```python
from build123d import *

# Parameters (mm, degrees)
CHAMFER1_SIZE      = 2.54
CUT_EXTRUDE1_DEPTH = 111.185656707
SKETCH6_R          = 58.335249529
SKETCH6_R_2        = 20.235249529
CUT_EXTRUDE2_DEPTH = 5.08
CUT_EXTRUDE3_START = -5.08
SKETCH7_R          = 58.335249529
SKETCH7_R_2        = 20.235249529
CUT_EXTRUDE3_DEPTH = 5.08
FILLET15_R         = 7.62


with BuildPart() as part:
    # Sketch2 → Revolve1 (revolve)
    with BuildSketch(Plane.YZ, mode=Mode.PRIVATE) as revolve1_sk:
        Polygon((8.128, 0), (8.128, 19.304), (76.708, 19.304), (76.708, 12.065), (64.008, 12.065), (64.008, 7.239), (76.708, 7.239), (76.708, 0), align=None)
    revolve(revolve1_sk.sketch.rotate(Axis((0, 0, 0), (0, 0, 1)), 90), axis=Axis((0, 0, 0), (0, 0, 1)))

    # Chamfer1
    chamfer1_edges = [part.edges().sort_by_distance(p)[0] for p in [
        (76.708, 0, 0),
        (76.708, 0, 7.239),
        (76.708, 0, 12.065),
        (76.708, 0, 19.304),
    ]]
    chamfer(chamfer1_edges, length=CHAMFER1_SIZE)

    # Sketch5 → Cut-Extrude1 (cut, through all)
    with BuildSketch(Plane(origin=(0, 0, 0), x_dir=(1, 0, 0), z_dir=(0, 0, -1))):
        with BuildLine():
            Line((-58.42, 0), (-20.32, 0))
            ThreePointArc((-20.32, 0), (-13.061444229, 15.566023084), (3.52853097, 20.011293541))
            Line((3.52853097, 20.011293541), (10.144526539, 57.532468931))
            ThreePointArc((10.144526539, 57.532468931), (-37.551652158, 44.752316367), (-58.42, 0))
        make_face()
        with BuildLine():
            Line((29.21, -50.593204089), (10.16, -17.597636205))
            ThreePointArc((10.16, -17.597636205), (-6.949849312, -19.094554054), (-19.094554054, -6.949849312))
            Line((-19.094554054, -6.949849312), (-54.896842906, -19.980816773))
            ThreePointArc((-54.896842906, -19.980816773), (-19.980816773, -54.896842906), (29.21, -50.593204089))
        make_face()
        with BuildLine():
            Line((15.5725915, -12.921289312), (44.68739374, -37.497175605))
            ThreePointArc((44.68739374, -37.497175605), (57.44900601, 10.129809775), (29.167624765, 50.519808029))
            Line((29.167624765, 50.519808029), (10.117624765, 17.524240144))
            ThreePointArc((10.117624765, 17.524240144), (19.918066395, 3.568746925), (15.5725915, -12.921289312))
        make_face()
    extrude(amount=-CUT_EXTRUDE1_DEPTH, mode=Mode.SUBTRACT)

    # Sketch6 → Cut-Extrude2 (cut)
    with BuildSketch(Plane(origin=(0, 0, 0), x_dir=(1, 0, 0), z_dir=(0, 0, -1))):
        Circle(SKETCH6_R)
        with Locations(Location((0, 0, 0), (0, 0, 60))):
            Circle(SKETCH6_R_2, mode=Mode.SUBTRACT)
    extrude(amount=-CUT_EXTRUDE2_DEPTH, mode=Mode.SUBTRACT)

    # Sketch7 → Cut-Extrude3 (cut)
    with BuildSketch(Plane(origin=(0, 0, 19.304), x_dir=(0, -1, 0), z_dir=(0, 0, 1)).offset(CUT_EXTRUDE3_START)):
        Circle(SKETCH7_R)
        with Locations(Location((0, 0, 0), (0, 0, 90))):
            Circle(SKETCH7_R_2, mode=Mode.SUBTRACT)
    extrude(amount=CUT_EXTRUDE3_DEPTH, mode=Mode.SUBTRACT)

    # Fillet15
    # the kernel refuses this fillet: 7.62 mm, written as the material it adds along each edge
    with BuildSketch(Plane(origin=(10.16, 17.597636205, 5.08), x_dir=(-0.9266160044504649, 0.3760090162433024, 0), z_dir=(0, 0, 1)), Plane(origin=(-20.32, 0, 5.08), x_dir=(0.13767464210654276, -0.9904775075289874, 0), z_dir=(0, 0, 1))) as fillet15_piece_1:
        with BuildLine():
            CenterArc((6.644178228, -7.547438607), FILLET15_R, 97.913310066, 74.173379868)
            Line((-0.903260379, -6.498357835), (0, 0))
            ThreePointArc((0, 0), (2.797548728, -0.193497047), (5.595097455, 0))
        make_face()
    extrude(amount=9.144)
    with BuildSketch(Plane(origin=(-19.094554054, 6.949849312, 5.08), x_dir=(0.4681351043427711, 0.8836569040538205, 0), z_dir=(0, 0, 1)), Plane(origin=(3.52853097, -20.011293541, 5.08), x_dir=(-0.9993368793115024, -0.03641155926279142, 0), z_dir=(0, 0, 1))) as fillet15_piece_2:
        with BuildLine():
            CenterArc((6.644178228, 7.547438607), FILLET15_R, 187.913310066, 74.173379868)
            Line((-0.903260379, 6.498357835), (0, 0))
            ThreePointArc((0, 0), (2.797548728, 0.193497047), (5.595097455, 0))
        make_face()
    extrude(amount=9.144)
    with BuildSketch(Plane(origin=(15.5725915, 12.921289312, 5.08), x_dir=(0.5270307863696181, -0.8498461920951471, 0), z_dir=(0, 0, 1))) as fillet15_piece_3:
        with BuildLine():
            CenterArc((6.592305904, 7.548065724), FILLET15_R, 188.362749939, 73.758264082)
            Line((-0.946671381, 6.439814174), (0, 0))
            ThreePointArc((0, 0), (2.773873375, 0.191024675), (5.54774675, 0))
        make_face()
    extrude(amount=9.144)
    with BuildSketch(Plane(origin=(10.117624765, -17.524240144, 5.08), x_dir=(0.5000000000000031, -0.8660254037844368, 0), z_dir=(0, 0, 1))) as fillet15_piece_4:
        with BuildLine():
            CenterArc((6.557483186, 7.62), FILLET15_R, 195.876042448, 74.123957552)
            ThreePointArc((-0.771857845, 5.535495248), (-0.193893401, 2.794524654), (0, 0))
            Line((0, 0), (6.557483186, 0))
        make_face()
    extrude(amount=9.144)


solid = part.part
```
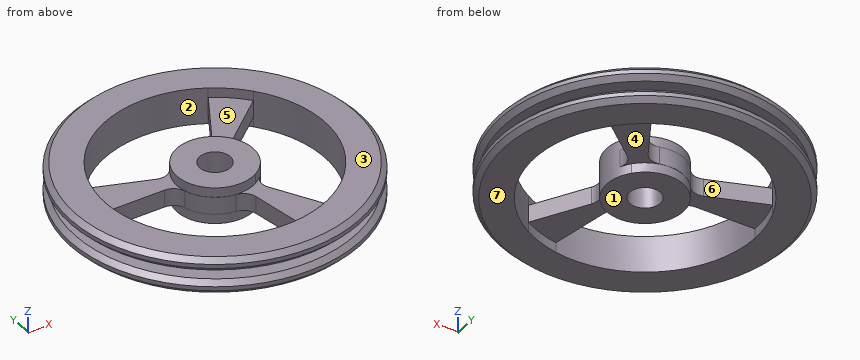
CAD build for the part. Positions are in the model's coordinates, mm. Face numbers are marked on the shaded views. A direction names the side the tool comes from. Round coordinates to 2 decimals unless told otherwise and drop trailing zeros. Return JSON: item names as keys, results as strings. Group by question number.
Item 1: Flat gauge pins, fed straight in: pin 1 Ø5 at (x, z) = (-34, 15.5) entering from +Y; pin 2 Ø2 at (y, z) = (32.5, 13) entering from +X; pin 3 Ø6 at (x, z) = (-36.5, 5.5) entering from -Y. Where does each tip first touch, or does it go through?
Item 2: Mould opens along X. For the marked faces 6 and 7 say: +X half, -X half, draft (parallel to the pull), parting line (faces both ways), or undercut.
Item 3: Probe probe 1 along Y at (x, z) = (0, 13); probe 2 along X at (y, z) = (30.5, 13.25); probe 3 along Z at (x, y) = (-44, 53.5) (3 decimals). List the from-to ranges inside material, lowest first.
Item 4: Band-saw the part on A-A on x = 0. State how many separate pieces and enclosed holes the cut face has, plus the area to 3 significant figures.
Item 5: 3-axis set-ups, long thin cutter, end or side, ignore diameter. For the marked faces 1, 2, 3, 4 and 5: which of +Z, -Z, +X, -X, +Y, -Y reach the whole face in a straight line?
Resolved:
{
 "1": {"pin 1": "stops at y = 69.94", "pin 2": "stops at x = 68.91", "pin 3": "stops at y = -68.95"},
 "2": {"face 6": "undercut", "face 7": "draft"},
 "3": {"probe 1": "y = -75.1 to -58.42, -20.72 to -8.13, 8.13 to 20.32, 58.42 to 75.1", "probe 2": "x = -68.9 to -49.83, 17.61 to 36.4, 49.73 to 68.9", "probe 3": "z = 0 to 7.239, 12.065 to 19.304"},
 "4": {"separate pieces": "4", "enclosed holes": "0", "area": "1,030 mm²"},
 "5": {"face 1": "-Z, +X, -X, +Y, -Y", "face 2": "+Z, -Z", "face 3": "+Z, +X, -X, +Y, -Y", "face 4": "-Z", "face 5": "+Z"}
}
